Work out the finished part from the listing and answer in its coordinate system (mm). Give positions to 0.01 mm unless a question says otherwise; leave off trailing zeros. Loops run counter-clockwise (first coordinate to the right, second up) from the corner with the lowest first, then second, coordinate; pieces in that order, holes last. Notation, with made-up numbers: M 2.5,-18 L 17.5,-18 A26 cw 17.5,13 Z; hole C -25.75,86.5 d4. An arc over 180 degrees is marked long. Write item = value, one per line. Start each with the question number.
1. Consider L1, parallel to X at y = 0, z = 11.7; L2, parallel to Y at x = 300, z = 12.5. Determine where each line is inside the solid, lowest interval first. Write a range as [from, to].
2. Flat-ended cylindrical pins translate along their axes: pin 1 Ø3 at (y, z) = (203.5, 9.5) entering from -X; pin 2 Ø9 at (x, y) = (299.5, -3.5) entering from -Z; pin 3 Ø5 at (y, z) = (-154, 8) entering from +X. Find the tip coordinate at first contact, or state that the pin passes through.
3. Section B-B on z = 4.5 is taken. Determine the outline of the cut face in (x, y).
4. Section A-A on x = 0 is taken. Determine the outline of the cut face in (y, z).
```python
from build123d import *

# Parameters (mm, degrees)
BOSS_EXTRUDE1_DEPTH = 15
FILLET1_R           = 10
BOSS_EXTRUDE2_START = -0.9999999999999974
SKETCH4_R           = 8.890000000000002
SKETCH4_R_2         = 8.890000000000008
SKETCH4_R_3         = 8.890000000000004
BOSS_EXTRUDE2_DEPTH = 0.9999999999999974


with BuildPart() as part:
    # Sketch2 → Boss-Extrude1 (new body)
    with BuildSketch(Plane.XY):
        with BuildLine():
            Line((0, 0), (-291.11000000000007, 0))
            ThreePointArc((-291.11000000000007, -2.18e-15), (-293.667421840922, -6.23943537983746), (-299.86827983333353, -8.889024119536039))
            ThreePointArc((-299.8682798333336, -8.88902411952966), (-5.91709e-12, -300.00000000000006), (299.86827983333325, -8.889024119541757))
            ThreePointArc((299.86827983333325, -8.889024119536035), (293.66742184092186, -6.23943537983736), (291.11000000000007, 1.09e-15))
            Line((291.1100000000001, 0), (0, 0))
        make_face()
        with BuildLine():
            ThreePointArc((-299.86827983333353, 8.889024119536039), (-293.667421840922, 6.23943537983746), (-291.11000000000007, 0))
            Line((-291.11000000000007, 0), (0, 0))
            Line((0, 0), (0, 291.11000000000007))
            ThreePointArc((1.0101e-13, 291.11000000000007), (-6.239435379837412, 293.6674218409219), (-8.889024119536034, 299.86827983333353))
            ThreePointArc((-8.889024119531676, 299.86827983333353), (-212.13203435596503, 212.13203435596358), (-299.8682798333336, 8.8890241195296))
        make_face()
        with BuildLine():
            Line((0, 291.11000000000007), (0, 0))
            Line((0, 0), (291.1100000000001, 0))
            ThreePointArc((291.11000000000007, 1.09e-15), (293.66742184092186, 6.239435379837364), (299.86827983333325, 8.889024119536035))
            ThreePointArc((299.86827983333325, 8.889024119541785), (212.1320343559607, 212.13203435596787), (8.889024119531646, 299.86827983333353))
            ThreePointArc((8.889024119536034, 299.86827983333353), (6.239435379837482, 293.66742184092203), (1.0101e-13, 291.11000000000007))
        make_face()
        with BuildLine():
            ThreePointArc((299.86827983333325, -8.889024119541757), (-5.91709e-12, -300.00000000000006), (-299.8682798333336, -8.88902411952966))
            ThreePointArc((-299.86827983333353, -8.889024119536039), (-306.2394353798375, -6.332578159078076), (-308.89000000000004, 1.09e-15))
            Line((-308.89000000000004, 0), (-350, 0))
            ThreePointArc((-350, 4.286e-14), (-6.429e-14, -350), (350, -8.573e-14))
            Line((350, 0), (308.8900000000001, 0))
            ThreePointArc((308.89000000000004, -2.18e-15), (306.2394353798374, -6.332578159078179), (299.86827983333325, -8.889024119536035))
        make_face()
        with BuildLine():
            ThreePointArc((8.889024119531646, 299.86827983333353), (212.1320343559607, 212.13203435596787), (299.86827983333325, 8.889024119541785))
            ThreePointArc((299.86827983333325, 8.889024119536035), (306.2394353798374, 6.332578159078173), (308.89000000000004, 0))
            Line((308.8900000000001, 0), (350, 0))
            ThreePointArc((350, 0), (247.48737341529164, 247.48737341529161), (9.915e-14, 350))
            Line((0, 350), (0, 308.89000000000004))
            ThreePointArc((9.924e-14, 308.89000000000004), (6.286179284748443, 306.2861792847484), (8.89, 300.00000000000006))
            ThreePointArc((8.89, 300.00000000000006), (8.889756026536256, 299.9341381091804), (8.889024119536034, 299.86827983333353))
        make_face()
        with BuildLine():
            ThreePointArc((-308.89000000000004, 1.09e-15), (-306.2394353798375, 6.332578159078078), (-299.86827983333353, 8.889024119536039))
            ThreePointArc((-299.8682798333336, 8.8890241195296), (-212.13203435596503, 212.13203435596358), (-8.889024119531676, 299.86827983333353))
            ThreePointArc((-8.889024119536034, 299.86827983333353), (-6.332578159078046, 306.2394353798375), (9.924e-14, 308.89000000000004))
            Line((0, 308.89000000000004), (0, 350))
            ThreePointArc((2.143e-14, 350), (-247.48737341529161, 247.48737341529164), (-350, 4.286e-14))
            Line((-350, 0), (-308.89000000000004, 0))
        make_face()
    extrude(amount=BOSS_EXTRUDE1_DEPTH)

    # Fillet1
    fillet1_edges = [part.edges().sort_by_distance(p)[0] for p in [
        (291.11000000000007, -3.375e-14, 0),
        (8.889024119535959, 300.13172016666664, 0),
        (-300.1317201666668, -8.889024119535831, 0),
        (-350, -1.4099e-13, 0),
    ]]
    fillet(fillet1_edges, radius=FILLET1_R)

    # Sketch4 → Boss-Extrude2 (add)
    with BuildSketch(Plane.XY.offset(15).offset(BOSS_EXTRUDE2_START)):
        with Locations((0, 300.00000000000006)):
            Circle(SKETCH4_R)
        with Locations((300.00000000000006, 0)):
            Circle(SKETCH4_R_2)
        with Locations((-300.00000000000006, 0)):
            Circle(SKETCH4_R_3)
    extrude(amount=BOSS_EXTRUDE2_DEPTH)


solid = part.part
```
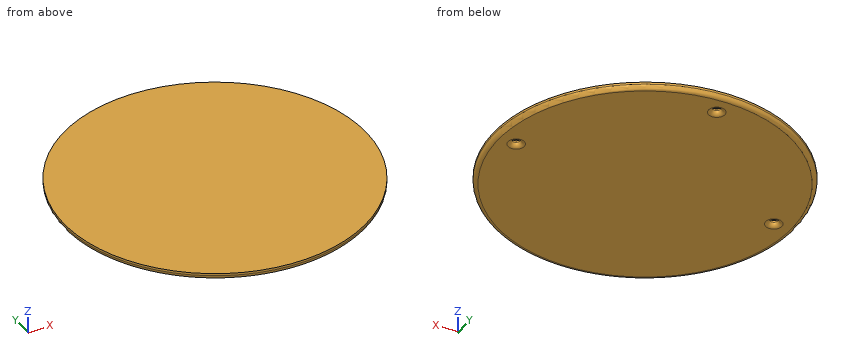
Verdict:
q1.L1 = [-350, -308.89], [-291.11, 291.11], [308.89, 350]
q1.L2 = [-180.28, -8.89], [8.89, 180.28]
q2.pin_1 = -285.81
q2.pin_2 = 14
q2.pin_3 = 315.37
q3.outline = C 0,0 d696.7; hole C -300,0 d21.08; hole C 0,300 d21.08; hole C 300,0 d21.08
q4.outline = M -350,10 A10 ccw -340,0 L 281.11,0 A10 ccw 291.11,10 L 291.11,14 L 308.89,14 L 308.89,10 A10 ccw 318.89,0 L 340,0 A10 ccw 350,10 L 350,15 L -350,15 Z
